from build123d import *

# Parameters (mm, degrees)
F1_DEPTH = 64
F2_DEPTH = 4
F0_W     = 3
F0_H     = 5.1
F3_DEPTH = 20


with BuildPart() as f1:
    # F0 (on Top) → F1 (new body)
    with BuildSketch(Plane.XY):
        with BuildLine():
            ThreePointArc((0, -35), (-24.748737, -24.748737), (-35, 0))
            Line((-35, 0), (-35, -38))
            Line((-35, -38), (-25.55, -38))
            Line((-25.55, -38), (-22.55, -38))
            Line((-22.55, -38), (0, -38))
            Line((0, -38), (0, -35))
        make_face()
        with BuildLine():
            Line((35, -38), (35, 0))
            ThreePointArc((35, 0), (24.748737, -24.748737), (0, -35))
            Line((0, -35), (0, -38))
            Line((0, -38), (22.55, -38))
            Line((22.55, -38), (25.55, -38))
            Line((25.55, -38), (35, -38))
        make_face()
    extrude(amount=F1_DEPTH)

    # F0 (on Top) → F2 (join)
    with BuildSketch(Plane.XY):
        Polygon((22.55, -38), (0, -38), (-22.55, -38), (-22.55, -43.1), (22.55, -43.1), align=None)
    extrude(amount=F2_DEPTH)

    # F0 (on Top) → F3 (join)
    with BuildSketch(Plane.XY):
        with Locations((-24.05, -40.55)):
            Rectangle(F0_W, F0_H)
        with Locations((24.05, -40.55)):
            Rectangle(F0_W, F0_H)
    extrude(amount=F3_DEPTH)


solid = f1.part
Work out the finished part from the listing and answer in its coordinate system (mm). A direction names the side the tool comes from. Give positions to 0.01 mm unless a question says otherwise; leave off trailing zeros. Loops run counter-clockwise (first coordinate to the right, second up) from the corner with the lowest first, then second, coordinate; pieces in that order, holes last. Notation, with made-up numbers: (24.5, 84.25) - (51.5, 84.25) arc R7 cw to (51.5, 89.25) - close; hole circle Ø8 at (44, 74). An arc over 180 degrees is marked (long way). Answer in a Markdown table with one row per item. Add a question column.
Q1. Determine the mould class of faces 1 (the flat face through (35, -19, 32)), 2 (the flat face through (-25.55, -41, 10)), 3 (the flat face through (22.55, -41, 12)), 4 (the flat face through (0, -36, 64)) for opening direction X: released by +X, released by -X, zero draft, split by the parting line, or undercut.
Q2. The part is cut by section B-B (z = 11.5). Determine the outline of the cut face in (x, y), and give its area (3 significant figures).
Q3. Each of these flat-tipped pins is pushed along its axis until it touches: P1, Ø1.5, axis at x = 23.5, y = -41.5, coming from the +Z side; P2, Ø10, axis at x = 5.5, y = -28, coming from the -Z side; P3, Ø4, axis at x = 1, z = 31, coming from the -Y side; P4, Ø1.5, axis at y = -39.5, z = 14.5, coming from the +X side. Where does it stop, or does it pass through?
Q4. Consider line 1 along Y through (x, z) = (-1, 38); line 2 along X through (y, z) = (-22.5, 7); line 3 along X through (y, z) = (-16.5, 18.5). Determine where each line is inside the solid, lowest interval first.
Q5. The part is cut by section C-C (y = -40). Determine the outline of the cut face in (x, z), and give its area (3 significant figures).
Q6. A tool of negligible diameter and unlimited length cuts with its end or side. For faces 5 (the flat face through (-24, -41, 20)), 6 (the flat face through (0, -41, 4)), 7 (the flat face through (25.55, -41, 10)), 8 (the flat face through (0, -43.1, 3)), from which of +Z, -Z, +X, -X, +Y, -Y can it reach the whole face along a straight path? Write none if from no direction.
Q7. The part is cut by section D-D (x = -28). Determine the outline of the cut face in (y, z).
Q8. The part is cut by section A-A (y = -28). Determine the outline of the cut face in (x, z).
Solution:
| question | item | result |
|---|---|---|
| 1 | face 1 | released by +X |
| 1 | face 2 | released by -X |
| 1 | face 3 | undercut |
| 1 | face 4 | zero draft |
| 2 | outline | (-35, -38) - (-25.55, -38) - (-25.55, -43.1) - (-22.55, -43.1) - (-22.55, -38) - (22.55, -38) - (22.55, -43.1) - (25.55, -43.1) - (25.55, -38) - (35, -38) - (35, 0) arc R35 cw to (0, -35) arc R35 cw to (-35, 0) - close |
| 2 | area | 766 mm² |
| 3 | P1 | stops at z = 20 |
| 3 | P2 | passes through |
| 3 | P3 | stops at y = -38 |
| 3 | P4 | stops at x = 25.55 |
| 4 | line 1 | y = -38 to -34.99 |
| 4 | line 2 | x = -35 to -26.81, 26.81 to 35 |
| 4 | line 3 | x = -35 to -30.87, 30.87 to 35 |
| 5 | outline | (-25.55, 0) - (25.55, 0) - (25.55, 20) - (22.55, 20) - (22.55, 4) - (-22.55, 4) - (-22.55, 20) - (-25.55, 20) - close |
| 5 | area | 300 mm² |
| 6 | face 5 | +Z, +X, -X, -Y |
| 6 | face 6 | +Z, -Y |
| 6 | face 7 | +Z, -Z, +X, -Y |
| 6 | face 8 | +Z, -Z, +X, -X, -Y |
| 7 | outline | (-38, 0) - (-21, 0) - (-21, 64) - (-38, 64) - close |
| 8 | outline | (-35, 0) - (-21, 0) - (-21, 64) - (-35, 64) - close; (21, 0) - (35, 0) - (35, 64) - (21, 64) - close |
